from build123d import *

# Parameters (mm, degrees)
F0_R     = 38.1
F1_DEPTH = 19.05
F2_R     = 31.75
F3_DEPTH = 19.05
F4_R     = 2.54
F5_R     = 2.54


with BuildPart() as f1:
    # F0 (on Front) → F1 (new body)
    with BuildSketch(Plane.XZ):
        Circle(F0_R)
    extrude(amount=F1_DEPTH)

    # F2 (on face) → F3 (cut, through all)
    with BuildSketch(Plane.XZ.offset(19.05)):
        Circle(F2_R)
    extrude(amount=-F3_DEPTH, mode=Mode.SUBTRACT)

    # F4
    f4_edges = [f1.edges().sort_by_distance(p)[0] for p in [
        (-38.1, -19.05, 0),
    ]]
    fillet(f4_edges, radius=F4_R)

    # F5
    f5_edges = [f1.edges().sort_by_distance(p)[0] for p in [
        (-31.75, -19.05, 0),
        (-38.1, 0, 0),
        (-31.75, 0, 0),
    ]]
    fillet(f5_edges, radius=F5_R)


solid = f1.part
CAD build for the part. Positions are in the model's coordinates, mm. Give positions to 0.01 mm unless a question says otherwise; leave off trailing zeros. Write each loop counter-clockwise with the first axis right and the second up, starting at its lowest first coordinate (ties: lowest second). Pieces come first, ordered by that corner, then holes. Notation, with made-up numbers: (74, 8) - (87, 8) arc R31 ccw to (87, 46) - close; hole circle Ø8 at (51.5, -22). An arc over 180 degrees is marked (long way). Put each result on its own line as item: value.
(1) Drop flat-ended pins along their axis: pin 1 Ø4 at (x, y) = (-18.5, -5.5) entering from +Z; pin 2 Ø4 at (y, z) = (-5, -20.5) entering from +X; pin 3 Ø3 at (x, y) = (-28, -13) entering from -Z. Give the stop position or say it passes through.
Working result:
pin 1: z = 34.34
pin 2: x = 33.31
pin 3: z = -27.37
(2) Wall check: L1, parallel to Z at x = 0, y = -9; L2, parallel to X at y = -3.25, z = 1; L3, parallel to Z at x = -3, y = -18. Give the ranges that are in metal, low to high.
Working result:
L1: -38.1 to -31.75, 31.75 to 38.1
L2: -38.09 to -31.73, 31.73 to 38.09
L3: -37.5 to -32.09, 32.09 to 37.5
(3) Saw through at B-B (z = 0). List the corners of the cut face in (x, y).
Working result:
outline: (-38.1, -16.51) arc R2.54 ccw to (-35.56, -19.05) - (-34.29, -19.05) arc R2.54 ccw to (-31.75, -16.51) - (-31.75, -2.54) arc R2.54 ccw to (-34.29, 0) - (-35.56, 0) arc R2.54 ccw to (-38.1, -2.54) - close; (31.75, -16.51) arc R2.54 ccw to (34.29, -19.05) - (35.56, -19.05) arc R2.54 ccw to (38.1, -16.51) - (38.1, -2.54) arc R2.54 ccw to (35.56, 0) - (34.29, 0) arc R2.54 ccw to (31.75, -2.54) - close
(4) Saw through at C-C (y = -8). List the corners of the cut face in (x, z), then the cut area to 3 significant figures.
Working result:
outline: circle Ø76.2 at (0, 0); hole circle Ø63.5 at (0, 0)
area: 1,390 mm^2
(5) Saw through at A-A (x = 0). List the corners of the cut face in (y, z).
Working result:
outline: (-19.05, -35.56) arc R2.54 ccw to (-16.51, -38.1) - (-2.54, -38.1) arc R2.54 ccw to (0, -35.56) - (0, -34.29) arc R2.54 ccw to (-2.54, -31.75) - (-16.51, -31.75) arc R2.54 ccw to (-19.05, -34.29) - close; (-19.05, 34.29) arc R2.54 ccw to (-16.51, 31.75) - (-2.54, 31.75) arc R2.54 ccw to (0, 34.29) - (0, 35.56) arc R2.54 ccw to (-2.54, 38.1) - (-16.51, 38.1) arc R2.54 ccw to (-19.05, 35.56) - close
(6) Pull direction X, two halves, no side cores. Call faces 1 (the flat face through (-19, -19.05, 29)), 2 (the cylindrical face through (-30.235, -9.427, -23.183)), 3 (the cylindrical face through (-6.883, -9.623, -30.995)): released by +X, released by -X, zero draft, split by the parting line, or undercut.
Working result:
face 1: zero draft
face 2: split by the parting line
face 3: undercut
